from build123d import *

# Parameters (mm, degrees)
F1_DEPTH = 25.4
F2_DEPTH = 76.2
F4_R     = 7.9375
F5_DEPTH = 12.7
F6_R     = 6.35
F7_R     = 6.35


with BuildPart() as f1:
    # F0 (on Front) → F1 (new body, symmetric)
    with BuildSketch(Plane.XZ):
        Polygon((26.5287997477, 235.5093256942), (-24.2712002523, 286.3093256942), (-24.2712002523, 235.5093256942), (-24.2712002523, -69.2906743058), (26.5287997477, -69.2906743058), align=None)
        Polygon((26.5287997477, 286.3093256942), (-24.2712002523, 286.3093256942), (26.5287997477, 235.5093256942), (166.2287997477, 235.5093256942), (166.2287997477, 286.3093256942), align=None)
    extrude(amount=F1_DEPTH, both=True)

    # F0 (on Front) → F2 (join, symmetric)
    with BuildSketch(Plane.XZ):
        Polygon((166.2287997477, 337.1093256942), (166.2287997477, 286.3093256942), (166.2287997477, 235.5093256942), (166.2287997477, 184.7093256942), (170.9912997477, 184.7093256942), (170.9912997477, 337.1093256942), align=None)
    extrude(amount=F2_DEPTH, both=True)

    # F4 (on offset) → F5 (cut, symmetric)
    with BuildSketch(Plane.YZ.offset(170.9912997477)):
        with Locations((0, 314.0905756942)):
            Circle(F4_R)
        with Locations((-50.5783743572, 277.3432357263)):
            Circle(F4_R)
        with Locations((-31.2591544485, 217.8847906621)):
            Circle(F4_R)
        with Locations((31.2591544485, 217.8847906621)):
            Circle(F4_R)
        with Locations((50.5783743572, 277.3432357263)):
            Circle(F4_R)
    extrude(amount=F5_DEPTH, both=True, mode=Mode.SUBTRACT)

    # F6
    f6_edges = [f1.edges().sort_by_distance(p)[0] for p in [
        (70.9788, -25.4, 286.309326),
        (70.9788, 25.4, 286.309326),
        (-24.2712, 0, 286.309326),
        (-24.2712, -25.4, 108.509326),
        (26.5288, -25.4, 83.109326),
        (26.5288, 25.4, 83.109326),
        (-24.2712, 25.4, 108.509326),
    ]]
    fillet(f6_edges, radius=F6_R)

    # F7
    f7_edges = [f1.edges().sort_by_distance(p)[0] for p in [
        (96.3788, -25.4, 235.509326),
        (96.3788, 25.4, 235.509326),
    ]]
    fillet(f7_edges, radius=F7_R)


solid = f1.part
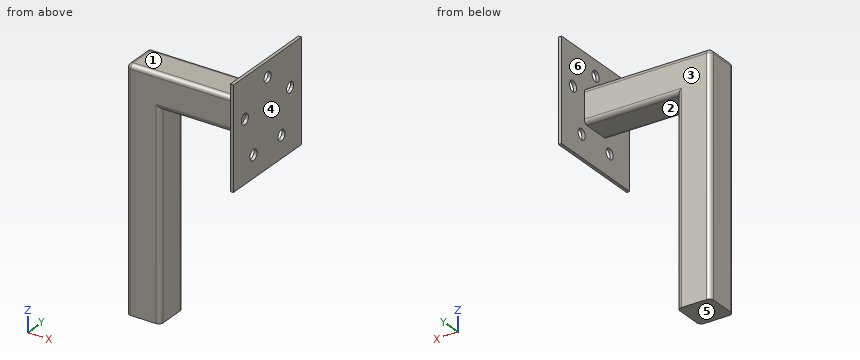
Geometry check sheet. Reference: the model listing, model coordinates, mm. Face numbers are marked on the shaded views. A direction names the side the tool comes from. Give positions to 0.01 mm unless a question says otherwise; leave off trailing zeros. Order: outer loops, then holes, each group sorted by start corner. A loop starts at its lowest first (then second) coordinate and runs counter-clockwise, first axis right, second up.
1. Sectioned sample at A-A (y = 0). Record the boundary of the cut face in (x, z), then the cut area to 3 significant figures.
Completed:
outline: (-24.27, -69.29) - (26.53, -69.29) - (26.53, 235.51) - (166.23, 235.51) - (166.23, 184.71) - (170.99, 184.71) - (170.99, 306.15) - (166.23, 306.15) - (166.23, 286.31) - (-17.92, 286.31) arc R6.35 ccw to (-24.27, 279.96) - close; (166.23, 322.03) - (170.99, 322.03) - (170.99, 337.11) - (166.23, 337.11) - close
area: 25,800 mm2
2. Draft check along X on the marked faces 4, 5 and 6. Enter one of: pulls with the +X half, pulls with the -X half, needs draft (parallel to the pull), parting line crosses it, or undercut.
Completed:
face 4: pulls with the +X half
face 5: needs draft
face 6: undercut
3. Access from +Z, -Z, +X, -X, +Y, -Y to the whole of each face (thin tool, end or side, straight path). Record for the marked faces 1, 2 and 3.
Completed:
face 1: +Z, -X, +Y, -Y
face 2: -Z, +Y, -Y
face 3: +Z, -Z, -X, +Y
4. Sectioned sample at C-C (x = 122). Record the boundary of the cut face in (y, z), then the cut area to 3 significant figures.
Completed:
outline: (-25.4, 241.86) arc R6.35 ccw to (-19.05, 235.51) - (19.05, 235.51) arc R6.35 ccw to (25.4, 241.86) - (25.4, 279.96) arc R6.35 ccw to (19.05, 286.31) - (-19.05, 286.31) arc R6.35 ccw to (-25.4, 279.96) - close
area: 2,550 mm2
5. Sectioned sample at B-B (z = -42). Record the boundary of the cut face in (x, y).
Completed:
outline: (-24.27, -19.05) arc R6.35 ccw to (-17.92, -25.4) - (20.18, -25.4) arc R6.35 ccw to (26.53, -19.05) - (26.53, 19.05) arc R6.35 ccw to (20.18, 25.4) - (-17.92, 25.4) arc R6.35 ccw to (-24.27, 19.05) - close
6. Sectioned sample at D-D (y = 48). Record the boundary of the cut face in (x, z).
Completed:
outline: (166.23, 184.71) - (170.99, 184.71) - (170.99, 269.84) - (166.23, 269.84) - close; (166.23, 284.85) - (170.99, 284.85) - (170.99, 337.11) - (166.23, 337.11) - close
7. Depth check by flat-ended pin: pin 1 (14.5 mm diameter, centred on y = 0, z = 314.09, fed in from -X); pin 2 (20.5 mm diameter, centred on y = 31.26, z = 217.88, fed in from +X); pin 3 (2.5 mm diameter, centred on x = 168, y = -13, fed in from -Z); pin 4 (18.5 mm diameter, centred on y = -31.26, z = 217.88, fed in from -X). Enter the tip coordinate at first touch or a pass-through.
Completed:
pin 1: passes through
pin 2: stops at x = 170.99
pin 3: stops at z = 184.71
pin 4: stops at x = -23.54
8. Scan lines: line 1 (X direction, y = 17, z = 186); line 2 (Z direction, x = 168.3, y = 0); line 3 (X direction, y = 28, z = 230). Record each from-to range of solid material in increasing order.
Completed:
line 1: x = -24.27 to 26.53, 166.23 to 170.99
line 2: z = 184.71 to 306.15, 322.03 to 337.11
line 3: x = 166.23 to 170.99
